Verification items for the finished model (mm, model axes). Face numbers are marked on the shaded views. A direction names the side the tool comes from. Give positions to 0.01 mm unless a question says otherwise; leave off trailing zeros. Loops run counter-clockwise (first coordinate to the right, second up) from the corner with the lowest first, then second, coordinate; pieces in that order, holes last. Notation, with made-up numbers: M 33,44 L 88,44 A36 cw 88,82 Z; hole C 9,43.5 d10. An arc over 180 degrees is marked long. Answer in a Markdown table with one row per item.
Autodesk Inventor part; units mm, degrees
ref_plane "Arbeitsebene2" through (-44.2034, 20.4204, 13.5) normal (0, 0, -1) x (0, 1, 0)
ref_plane "YZ Plane" through (0, 0, 0) normal (1, 0, 0) x (0, 1, 0)
ref_plane "XZ Plane" through (0, 0, 0) normal (0, 1, 0) x (-1, 0, 0)
ref_plane "Arbeitsebene1" through (0, 0, 0) normal (0, 0, 1) x (1, 0, 0)
sketch "Skizze1" plane through (0, 0, 0) normal (0, 0, 1) x (1, 0, 0)
  line L0 (-69.421, 36.3204) -> (-72.421, 39.3204)
  line L1 (-69.421, 36.3204) -> (-60.421, 36.3204)
  line L2 (-57.421, 33.3204) -> (-60.421, 36.3204)
  line L3 (-57.421, 33.3204) -> (-57.421, -36.5796)
  line L4 (-60.421, -39.5796) -> (-57.421, -36.5796)
  line L5 (-60.421, -39.5796) -> (-69.421, -39.5796)
  line L6 (-72.421, -42.5796) -> (-69.421, -39.5796)
  line L7 (-72.421, -42.5796) -> (-72.421, -47.4152)
  arc A0 (-72.421, -47.4152) -> (-68.421, -51.4152) centre (-68.421, -47.4152) ccw
  line L8 (-68.421, -51.4152) -> (68.421, -51.4152)
  arc A1 (68.421, -51.4152) -> (72.421, -47.4152) centre (68.421, -47.4152) ccw
  line L9 (72.421, -47.4152) -> (72.421, -42.5796)
  line L10 (69.421, -39.5796) -> (72.421, -42.5796)
  line L11 (69.421, -39.5796) -> (65.421, -39.5796)
  line L12 (62.421, -36.5796) -> (65.421, -39.5796)
  line L13 (62.421, -36.5796) -> (62.421, 33.3204)
  line L14 (65.421, 36.3204) -> (62.421, 33.3204)
  line L15 (65.421, 36.3204) -> (69.421, 36.3204)
  line L16 (72.421, 39.3204) -> (69.421, 36.3204)
  line L17 (72.421, 39.3204) -> (72.421, 47.4152)
  arc A2 (72.421, 47.4152) -> (68.421, 51.4152) centre (68.421, 47.4152) ccw
  line L18 (68.421, 51.4152) -> (-68.421, 51.4152)
  arc A3 (-68.421, 51.4152) -> (-72.421, 47.4152) centre (-68.421, 47.4152) ccw
  line L19 (-72.421, 47.4152) -> (-72.421, 39.3204)
  circle A4 centre (68.921, 47.9152) radius 1.4
  circle A5 centre (68.921, -47.9152) radius 1.4
  circle A6 centre (-68.921, -47.9152) radius 1.4
  circle A7 centre (-68.921, 47.9152) radius 1.5
  circle A8 centre (-38.7933, -44.5796) radius 1.4
  circle A9 centre (-38.7933, 41.3204) radius 1.4
  line L20 (-48.1034, 36.3204) -> (-38.1034, 36.3204)
  line L21 (-38.1034, 36.3204) -> (-38.1034, -39.5796)
  line L22 (-38.1034, -39.5796) -> (-48.1034, -39.5796)
  line L23 (-48.1034, -39.5796) -> (-48.1034, 36.3204)
  circle A10 centre (-20.0933, 41.3204) radius 1.4
  circle A11 centre (-20.0933, -44.5796) radius 1.4
  line L24 (-19.4034, -39.5796) -> (-29.4034, -39.5796)
  line L25 (-29.4034, -39.5796) -> (-29.4034, 36.3204)
  line L26 (-29.4034, 36.3204) -> (-19.4034, 36.3204)
  line L27 (-19.4034, 36.3204) -> (-19.4034, -39.5796)
  circle A12 centre (-1.3933, 41.3204) radius 1.4
  circle A13 centre (-1.3933, -44.5796) radius 1.4
  line L28 (-0.7034, -39.5796) -> (-10.7034, -39.5796)
  line L29 (-10.7034, -39.5796) -> (-10.7034, 36.3204)
  line L30 (-10.7034, 36.3204) -> (-0.7034, 36.3204)
  line L31 (-0.7034, 36.3204) -> (-0.7034, -39.5796)
  circle A14 centre (17.3067, 41.3204) radius 1.4
  circle A15 centre (17.3067, -44.5796) radius 1.4
  line L32 (17.9966, -39.5796) -> (7.9966, -39.5796)
  line L33 (7.9966, -39.5796) -> (7.9966, 36.3204)
  line L34 (7.9966, 36.3204) -> (17.9966, 36.3204)
  line L35 (17.9966, 36.3204) -> (17.9966, -39.5796)
  circle A16 centre (36.0067, 41.3204) radius 1.4
  circle A17 centre (36.0067, -44.5796) radius 1.4
  line L36 (36.6966, -39.5796) -> (26.6966, -39.5796)
  line L37 (26.6966, -39.5796) -> (26.6966, 36.3204)
  line L38 (26.6966, 36.3204) -> (36.6966, 36.3204)
  line L39 (36.6966, 36.3204) -> (36.6966, -39.5796)
  circle A18 centre (54.7067, 41.3204) radius 1.4
  circle A19 centre (54.7067, -44.5796) radius 1.4
  line L40 (55.3966, -39.5796) -> (45.3966, -39.5796)
  line L41 (45.3966, -39.5796) -> (45.3966, 36.3204)
  line L42 (45.3966, 36.3204) -> (55.3966, 36.3204)
  line L43 (55.3966, 36.3204) -> (55.3966, -39.5796)
  line L44 (-32.7933, 44.3204) -> (-41.7933, 44.3204)
  line L45 (-41.7933, 44.3204) -> (-41.7933, -47.5796)
  line L46 (-41.7933, -47.5796) -> (-32.7933, -47.5796)
  line L47 (-32.7933, -47.5796) -> (-32.7933, 44.3204)
  circle A20 centre (-37.2933, 36.3204) radius 1.4
  circle A21 centre (-37.2933, -39.5796) radius 1.4
  point P0 (0, 0)
  dimension "d0" = 3
  dimension "d1" = 3
  dimension "d2" = 3
  dimension "d3" = 6
  dimension "d4" = 2.8
  dimension "d5" = 2.8
ref_plane "Arbeitsebene2" through (-44.2034, 20.4204, 13.5) normal (0, 0, -1) x (0, 1, 0)
extrude "Extrusion1" add sketch "Skizze1" along normal up to surface (13.5 mm away) contours L45 L44 L47 L46 L22 A21 L21 A20 L20 | L20 A20 L21 A21 L22 L45
sketch "Skizze2" plane through (-41.7933, -47.5796, 13.5) normal (0, 0, 1) x (1, 0, 0)
  line L0 (9, 68) -> (-3, 68)
  line L1 (-3, 80) -> (9, 80)
  line L2 (-3, 61.3) -> (9, 61.3)
  line L3 (9, 49.3) -> (-3, 49.3)
  line L4 (-3, 42.6) -> (9, 42.6)
  line L5 (9, 30.6) -> (-3, 30.6)
  line L6 (-3, 23.9) -> (9, 23.9)
  line L7 (9, 11.9) -> (-3, 11.9)
  line L8 (9, 80) -> (-3, 80)
  line L9 (-3, 80) -> (-3, 68)
  line L10 (-3, 68) -> (9, 68)
  line L11 (9, 68) -> (9, 80)
  line L12 (-3.2, 67.8) -> (-3.2, 80.2)
  line L13 (-3.2, 80.2) -> (9.2, 80.2)
  line L14 (9.2, 80.2) -> (9.2, 67.8)
  line L15 (9.2, 67.8) -> (-3.2, 67.8)
  point P0 (41.7933, 47.5796)
  dimension "d8" = 0.2
extrude "Extrusion2" cut sketch "Skizze2" against normal blind 2 contours L0 L9 L1 L11 | L12 L13 L14 L15
pattern_linear "Rechteckige Anordnung1" count 5 spacing 18.7 along (0, -1, 0) of "Extrusion2"
sketch "Skizze3" plane through (-41.7933, 20.2204, 13.5) normal (0, 0, 1) x (1, 0, 0)
  line L0 (0, -6.3) -> (9, -6.3)
  line L1 (9, -6.3) -> (9, 0)
  line L2 (9, 0) -> (0, 0)
  line L3 (0, 0) -> (0, -6.3)
  line L4 (0, -25) -> (9, -25)
  line L5 (9, -25) -> (9, -18.7)
  line L6 (9, -18.7) -> (0, -18.7)
  line L7 (0, -18.7) -> (0, -25)
  line L8 (0, -43.7) -> (9, -43.7)
  line L9 (9, -43.7) -> (9, -37.4)
  line L10 (9, -37.4) -> (0, -37.4)
  line L11 (0, -37.4) -> (0, -43.7)
  circle A0 centre (4.5, -3.15) radius 1.4
  circle A1 centre (4.5, -21.85) radius 1.4
  circle A2 centre (4.5, -40.55) radius 1.4
  point P0 (41.7933, -20.2204)
  dimension "d14" = 2.8
  dimension "d15" = 2.8
  dimension "d16" = 2.8
extrude "Extrusion3" cut sketch "Skizze3" against normal through all contours A0 | A1 | A2
sketch "Skizze4" plane through (-41.7933, -42.1796, 13.5) normal (0, 0, 1) x (1, 0, 0)
  circle A0 centre (3, 83.5) radius 1.4
  circle A1 centre (4.5, 78.5) radius 1.4
  line L0 (0, 74.8) -> (9, 74.8)
  line L1 (9, 74.8) -> (9, 86.5)
  line L2 (9, 86.5) -> (0, 86.5)
  line L3 (0, 86.5) -> (0, 74.8)
  line L4 (9, 0) -> (9, -5.4)
  line L5 (0, 0) -> (9, 0)
  line L6 (0, -5.4) -> (0, 0)
  line L7 (9, -5.4) -> (0, -5.4)
  circle A2 centre (3, -2.4) radius 1.4
  point P0 (41.7933, 42.1796)
hole "Bohrung1" at (-38.7933, 41.3204, 13.5) at (-38.7933, -44.5796, 13.5) direction (0, 0, -1) diameter 3.2 end through all counterbore diameter 7 counterbore depth 9
properties part number "Omniscope_USBC_Bar"
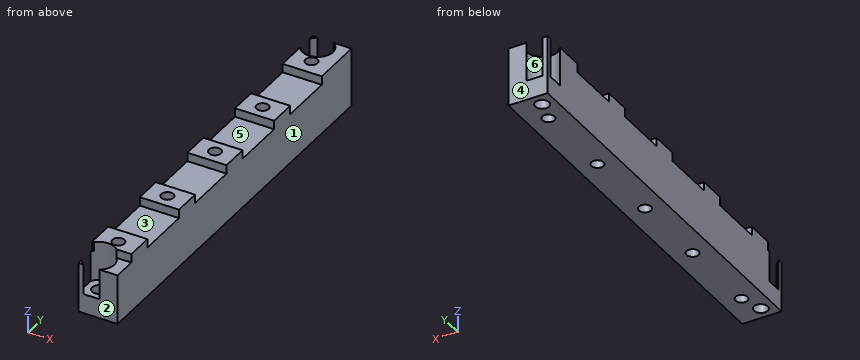
Item 1: Release check for a two-part mould opening along Y. For the marked faces 1, 2 and 3 record: released by +Y, released by -Y, zero draft, split by the parting line, or undercut.
Reported:
| item | result |
|---|---|
| face 1 | zero draft |
| face 2 | released by -Y |
| face 3 | undercut |
Item 2: Scan lines: L1, parallel to Y at x = -33.25, z = 12.25; L2, parallel to Y at x = -39, z = 13; L3, parallel to Y at x = -37.5, z = 8.75. Record each from-to range of solid material in increasing order. Write a range as [from, to].
Reported:
| item | result |
|---|---|
| L1 | y = [-42.18, -35.88], [-23.48, -17.18], [-4.78, 1.52], [13.92, 20.22], [32.62, 44.32] |
| L2 | y = [-41.09, -35.88], [-23.48, -17.18], [-4.78, 1.52], [13.92, 20.22], [32.62, 37.83] |
| L3 | y = [-41.33, -40.96], [-38.19, -21.71], [-18.94, -3.01], [-0.24, 15.69], [18.46, 34.94], [37.71, 38.07] |
Item 3: Sectioned sample at D-D (y = 26). Record the cut outline in (x, z).
Reported:
| item | result |
|---|---|
| outline | M -41.79,0 L -32.79,0 L -32.79,11.5 L -41.79,11.5 Z |
Item 4: Go/stop test with flat-tipped pins: pin 1 (3.5 mm diameter, centred on x = -35.5, y = -45.5, fed in from +Z); pin 2 (1.6 mm diameter, centred on x = -35.5, z = 12.5, fed in from -Y); pin 3 (3 mm diameter, centred on x = -38, y = -45, fed in from +Z); pin 4 (2 mm diameter, centred on x = -37.29, y = -20.33, fed in from +Z). Record where each tip stops, or that it passes through.
Reported:
| item | result |
|---|---|
| pin 1 | stops at z = 11.5 |
| pin 2 | stops at y = -42.18 |
| pin 3 | stops at z = 4.5 |
| pin 4 | passes through |
Item 5: Sectioned sample at B-B (x = -33.75). Record the cut outline in (y, z), and give its area (3 significant figures).
Reported:
| item | result |
|---|---|
| outline | M -47.58,0 L 44.32,0 L 44.32,13.5 L 32.62,13.5 L 32.62,11.5 L 20.22,11.5 L 20.22,13.5 L 13.92,13.5 L 13.92,11.5 L 1.52,11.5 L 1.52,13.5 L -4.78,13.5 L -4.78,11.5 L -17.18,11.5 L -17.18,13.5 L -23.48,13.5 L -23.48,11.5 L -35.88,11.5 L -35.88,13.5 L -42.18,13.5 L -42.18,11.5 L -47.58,11.5 Z |
| area | 1,130 mm^2 |
Item 6: Sectioned sample at A-A (z = 10.5). Record the cut outline in (x, y), and give its area (3 significant figures).
Reported:
| item | result |
|---|---|
| outline | M -41.79,-47.58 L -40.6,-47.58 A3.5 cw -41.79,-46.38 Z; M -41.79,-42.78 A3.5 cw long -36.99,-47.58 L -32.79,-47.58 L -32.79,44.32 L -36.99,44.32 A3.5 cw long -41.79,39.52 Z; M -41.79,43.12 A3.5 cw -40.6,44.32 L -41.79,44.32 Z; hole C -37.29,-39.58 d2.8; hole C -37.29,-20.33 d2.8; hole C -37.29,-1.63 d2.8; hole C -37.29,17.07 d2.8; hole C -37.29,36.32 d2.8 |
| area | 724 mm^2 |
Item 7: Tool access check on the marked faces 4, 5 and 6. Record the directions out of +Z, -Z, +X, -X, +Y, -Y that give a thin tool (end or side, any length) a straight path to the whole face; none if there is none.
Reported:
| item | result |
|---|---|
| face 4 | +Z, -Z, +X, -X, +Y |
| face 5 | +Z, +X, -X |
| face 6 | +Z |
Item 8: Sectioned sample at C-C (z = 3.25). Record the cut outline in (x, y).
Reported:
| item | result |
|---|---|
| outline | M -41.79,-47.58 L -32.79,-47.58 L -32.79,44.32 L -41.79,44.32 Z; hole C -38.79,-44.58 d3.2; hole C -38.79,41.32 d3.2; hole C -37.29,-39.58 d2.8; hole C -37.29,-20.33 d2.8; hole C -37.29,-1.63 d2.8; hole C -37.29,17.07 d2.8; hole C -37.29,36.32 d2.8 |
